Check sheet for the modelled part. Datum: model origin and axes. Units: mm. A direction names the side the tool comes from. Round coordinates to 2 decimals unless told otherwise and drop trailing zeros. Order: outer loops, then holes, each group sorted by start corner. A loop starts at its lowest first (then second) coordinate and runs counter-clockwise, first axis right, second up.
Q1. Depth check by flat-ended pin: P1, Ø8, axis at x = -12.5, z = -23.5, coming from the +Y side. Enter the tip coordinate at first touch or a pass-through.
Q2. Cross-section at A-A on y = 25. Record the cut outline in (x, z).
Q3. Set-up check for faces 1 (the flat face through (23.896, 15, -15)), 2 (the flat face through (3, 28.37, -29)): record each of +Z, -Z, +X, -X, +Y, -Y from which the full face is reachable in a straight line by a thin tool's end or side.
Q4. Mould release check, pull along X, two halves, no side actions. Record for faces 3 (the flat face through (-33.121, 14, -15)), 4 (the flat face through (31.621, 15, -15)), 5 (the flat face through (0, 14, 0)), 6 (the flat face through (33.121, 14, -15)): +X half, -X half, draft (parallel to the pull), parting line (faces both ways), or undercut.
Q5. Cross-section at C-C on x = 18.5. Record the cut outline in (y, z).
Q6. Scan lines: probe 1 along X at (y, z) = (11, -14); probe 2 along Z at (x, y) = (16, 22.75); probe 3 along Y at (x, z) = (-2, -17.25). Record each from-to range of solid material in increasing order.
Q7. Cross-section at B-B on z = -23. Record the cut outline in (x, y).
from build123d import *

# Parameters (mm, degrees)
F0_W     = 57.017289
F0_H     = 28.369613
F1_DEPTH = 29.718
F2_T     = -1.5


with BuildPart() as f1:
    # F0 (on Top) → F1 (new body)
    with BuildSketch(Plane.XY):
        with Locations((-4.612352, 14.184806)):
            Rectangle(F0_W, F0_H)
    extrude(amount=-F1_DEPTH)

    # F2
    f2_openings = [f1.faces().sort_by_distance(p)[0] for p in [
        (-4.612353, 28.369613, -14.859),
    ]]
    offset(amount=F2_T, openings=f2_openings)

    # F3: F1 across plane


with BuildPart() as f1_1:
    add(f1.part)
    add(f1.part.mirror(Plane.YZ))


solid = f1_1.part
Results found:
1. P1: stops at y = 1.5
2. outline: (-33.12, -29.72) - (33.12, -29.72) - (33.12, 0) - (-33.12, 0) - close; hole (-31.62, -28.22) - (-23.9, -28.22) - (-23.9, -1.5) - (-31.62, -1.5) - close; hole (-22.4, -28.22) - (22.4, -28.22) - (22.4, -1.5) - (-22.4, -1.5) - close; hole (23.9, -28.22) - (31.62, -28.22) - (31.62, -1.5) - (23.9, -1.5) - close
3. face 1: +Y
3. face 2: +Z, -Z, +X, -X, +Y
4. face 3: -X half
4. face 4: undercut
4. face 5: draft
4. face 6: +X half
5. outline: (0, -29.72) - (28.37, -29.72) - (28.37, -28.22) - (1.5, -28.22) - (1.5, -1.5) - (28.37, -1.5) - (28.37, 0) - (0, 0) - close
6. probe 1: x = -33.12 to -31.62, -23.9 to -22.4, 22.4 to 23.9, 31.62 to 33.12
6. probe 2: z = -29.72 to -28.22, -1.5 to 0
6. probe 3: y = 0 to 1.5
7. outline: (-33.12, 0) - (33.12, 0) - (33.12, 28.37) - (31.62, 28.37) - (31.62, 1.5) - (23.9, 1.5) - (23.9, 28.37) - (22.4, 28.37) - (22.4, 1.5) - (-22.4, 1.5) - (-22.4, 28.37) - (-23.9, 28.37) - (-23.9, 1.5) - (-31.62, 1.5) - (-31.62, 28.37) - (-33.12, 28.37) - close
